Design review of the part built by this model. Coordinates are the model's own, in mm. A direction names the side the tool comes from. Coordinates: 2 decimals unless noted, no trailing zeros. Write each loop counter-clockwise with the first axis right and the second up, starting at its lowest first coordinate (ties: lowest second). Pieces come first, ordered by that corner, then holes.
Q1. Add section A-A, the plane y = -49. Give the boundary of the cut face in (x, z).
Q2. Add section C-C, the plane y = 10.5. Give the boundary of the cut face in (x, z).
Q3. The part is to be moulded in two halves that separate along Z. For faces 5 (the face through (34, -52, -2.5)), 6 (the face through (0, -57.25, -32)), 7 (the face through (-34, -52, -2.5)), 8 (the face through (0.82, 54.77, -39.99)), say which applies: +Z half, -Z half, draft (parallel to the pull), parting line (faces both ways), or undercut.
Q4. Add section B-B, the plane x = 0. Give the boundary of the cut face in (y, z).
Q5. Machinability: for faces 1 (the face through (35.77, -1.24, -11.26)), 2 (the face through (35, 40.25, 0)), 3 (the face through (-34, -52, 2.5)), 4 (the face through (-35, 49, -4)), which of the approach directions +Z, -Z, +X, -X, +Y, -Y give a long, thin tool a straight path to every point of the face, cutting with its end or side? Answer none if there is none.
Q6. Clearance check with flat-ended pins moving along their axes: pin 1 Ø6 at (x, y) = (-35, -51.5) entering from -Z; pin 2 Ø2.5 at (x, z) = (34.5, -0.5) entering from +Y; pin 3 Ø3 at (x, y) = (-15, -36.5) entering from -Z. State where each tip first meets the part, or that it passes through.
Q7. To check wall thickness, follow probe 1 along X at (y, z) = (33, 0); probe 2 along X at (y, z) = (27, -2.5). State the ranges of each line that lie inside material, in increasing order.
Q8. Add section D-D, the plane y = 48. Give the boundary of the cut face in (x, z), plus the area to 3 significant figures.
from build123d import *

# Parameters (mm, degrees)
SKETCH1_R           = 37.5
SKETCH1_R_2         = 30
BOSS_EXTRUDE1_DEPTH = 57.25
SKETCH2_R           = 40
SKETCH2_R_2         = 37.5
BOSS_EXTRUDE2_DEPTH = 5
SKETCH3_W           = 90
SKETCH3_H           = 5
CUT_EXTRUDE1_DEPTH  = 10
CUT_EXTRUDE2_DEPTH  = 17
CHAMFER1_SIZE       = 1


with BuildPart() as part:
    # Sketch1 → Boss-Extrude1 (new body, symmetric)
    with BuildSketch(Plane(origin=(0, 0, 0), x_dir=(1, 0, 0), z_dir=(0, 1, 0))):
        Circle(SKETCH1_R)
        Circle(SKETCH1_R_2, mode=Mode.SUBTRACT)
    extrude(amount=BOSS_EXTRUDE1_DEPTH, both=True)

    # Sketch2 → Boss-Extrude2 (add)
    with BuildSketch(Plane(origin=(0, 57.25, 0), x_dir=(1, 0, 0), z_dir=(0, 1, 0))):
        Circle(SKETCH2_R)
        Circle(SKETCH2_R_2, mode=Mode.SUBTRACT)
    extrude(amount=-BOSS_EXTRUDE2_DEPTH)

    # Sketch3 → Cut-Extrude1 (cut)
    with BuildSketch(Plane.XZ.offset(57.25)):
        Rectangle(SKETCH3_W, SKETCH3_H)
    extrude(amount=-CUT_EXTRUDE1_DEPTH, mode=Mode.SUBTRACT)

    # Sketch4 → Cut-Extrude2 (cut)
    with BuildSketch(Plane(origin=(0, 57.25, 0), x_dir=(1, 0, 0), z_dir=(0, 1, 0))):
        with BuildLine():
            Line((32.756678708, -4), (39.799497484, -4))
            ThreePointArc((39.799497484, -4), (39.949842924, -2.002511002), (40, 0))
            ThreePointArc((40, 0), (39.949842924, 2.002511002), (39.799497484, 4))
            Line((39.799497484, 4), (32.756678708, 4))
            ThreePointArc((32.756678708, 4), (32.939113508, 2.003696911), (33, 0))
            ThreePointArc((33, 0), (32.939113508, -2.003696911), (32.756678708, -4))
        make_face()
        with BuildLine():
            ThreePointArc((-39.799497484, 4), (-40, 0), (-39.799497484, -4))
            Line((-39.799497484, -4), (-32.756678708, -4))
            ThreePointArc((-32.756678708, -4), (-33, 0), (-32.756678708, 4))
            Line((-32.756678708, 4), (-39.799497484, 4))
        make_face()
    extrude(amount=-CUT_EXTRUDE2_DEPTH, mode=Mode.SUBTRACT)

    # Chamfer1
    chamfer1_edges = [part.edges().sort_by_distance(p)[0] for p in [
        (0, 57.25, 40),
        (-30, 57.25, 0),
        (0, -57.25, -30),
        (0, -57.25, 30),
        (0, -57.25, -37.5),
        (0, -57.25, 37.5),
        (0, 52.25, -40),
        (0, 52.25, 40),
        (0, 57.25, -40),
    ]]
    chamfer(chamfer1_edges, length=CHAMFER1_SIZE)


solid = part.part
Here are the results:
1. outline: (-37.42, -2.5) arc R37.5 ccw to (37.42, -2.5) - (29.9, -2.5) arc R30 cw to (-29.9, -2.5) - close; (-37.42, 2.5) - (-29.9, 2.5) arc R30 cw to (29.9, 2.5) - (37.42, 2.5) arc R37.5 ccw to start
2. outline: circle Ø75 at (0, 0); hole circle Ø60 at (0, 0)
3. face 5: undercut
3. face 6: draft
3. face 7: undercut
3. face 8: -Z half
4. outline: (-57.25, -36.5) - (-56.25, -37.5) - (52.25, -37.5) - (52.25, -39) - (53.25, -40) - (56.25, -40) - (57.25, -39) - (57.25, -31) - (56.25, -30) - (-56.25, -30) - (-57.25, -31) - close; (-57.25, 31) - (-56.25, 30) - (56.25, 30) - (57.25, 31) - (57.25, 39) - (56.25, 40) - (53.25, 40) - (52.25, 39) - (52.25, 37.5) - (-56.25, 37.5) - (-57.25, 36.5) - close
5. face 1: -Y
5. face 2: +X, +Y
5. face 3: +X, -X, -Y
5. face 4: -X, +Y
6. pin 1: stops at z = -19.55
6. pin 2: stops at y = 40.25
6. pin 3: stops at z = -34.99
7. probe 1: x = -37.5 to -30, 30 to 37.5
7. probe 2: x = -37.42 to -29.9, 29.9 to 37.42
8. outline: (-37.29, -4) arc R37.5 ccw to (37.29, -4) - (32.76, -4) arc R33 ccw to (32.76, 4) - (37.29, 4) arc R37.5 ccw to (-37.29, 4) - (-32.76, 4) arc R33 ccw to (-32.76, -4) - close; hole circle Ø60 at (0, 0)
8. area: 1,520 mm2
